from build123d import *

# Parameters (mm, degrees)
SKETCH_1_W          = 35
SKETCH_1_H          = 39
SKETCH_1_R          = 2.1
EXTRUDE_1_DEPTH     = 8
SKETCH_2_R          = 1.6
CUT_EXTRUDE_1_DEPTH = 54.009433123
SKETCH_5_R          = 6
EXTRUDE_3_DEPTH     = 8
M4X0_7_1_D          = 3.3


with BuildPart() as part:
    # 草图1 → 凸台-拉伸1 (new body)
    with BuildSketch(Plane.XY):
        with Locations((17.5, 19.5)):
            Rectangle(SKETCH_1_W, SKETCH_1_H)
        with Locations((17.5, 23.5)):
            Circle(SKETCH_1_R, mode=Mode.SUBTRACT)
    extrude(amount=EXTRUDE_1_DEPTH)

    # 草图2 → 切除-拉伸1 (cut, through all)
    with BuildSketch(Plane(origin=(0, 39, 0), x_dir=(1, 0, 0), z_dir=(0, 1, 0))):
        with Locations(Location((5, -4, 0), (0, 0, 270))):
            Circle(SKETCH_2_R)
        with Locations(Location((30, -4, 0), (0, 0, 270))):
            Circle(SKETCH_2_R)
    extrude(amount=-CUT_EXTRUDE_1_DEPTH, mode=Mode.SUBTRACT)

    # 草图5 → 凸台-拉伸3 (add)
    with BuildSketch(Plane.XY.offset(8)):
        with BuildLine():
            Line((35, 39), (59.879399185, 32.179773011))
            ThreePointArc((59.879399185, 32.179773011), (66.424469933, 24.663544764), (62.025315767, 15.720442351))
            Line((62.025315767, 15.720442351), (35, 0))
            Line((35, 0), (35, 39))
        make_face()
        with Locations((57.5, 23.5)):
            Circle(SKETCH_5_R, mode=Mode.SUBTRACT)
    extrude(amount=-EXTRUDE_3_DEPTH)

    # M4x0.7 螺纹孔1 (through all)
    with Locations(Plane(origin=(0, 39, 0), x_dir=(1, 0, 0), z_dir=(0, 1, 0))):
        with Locations((5, -4), (30, -4)):
            Hole(M4X0_7_1_D / 2)


solid = part.part
CAD build for the part. Positions are in the model's coordinates, mm. Round coordinates to 2 decimals unless told otherwise and drop trailing zeros. Order: outer loops, then holes, each group sorted by start corner. A loop starts at its lowest first (then second) coordinate and runs counter-clockwise, first axis right, second up. Notation, with made-up numbers: (18, 13) -> (47, 13) arc R16 ccw to (47, 30) -> close; hole circle Ø7 at (58, 26.5). An arc over 180 degrees is marked (long way). Write each question's results on one line, items separated by ' | '.
1. Wall check: line 1 along X through (y, z) = (11.5, 4); line 2 along X through (y, z) = (21, 3.5); line 3 along X through (y, z) = (19.5, 4). Give the ranges that are in metal, low to high. Write a range as [from, to].
Findings below:
line 1: x = [0, 3.35], [6.65, 28.35], [31.65, 54.77] | line 2: x = [0, 3.43], [6.57, 28.43], [31.57, 52.05], [62.95, 66.15] | line 3: x = [0, 3.35], [6.65, 28.35], [31.65, 53.03], [61.97, 65.56]
2. Cut at D-D (x = 30). Give the cut face in (y, z).
Findings below:
outline: (0, 0) -> (39, 0) -> (39, 2.35) -> (0, 2.35) -> close; (0, 5.65) -> (39, 5.65) -> (39, 8) -> (0, 8) -> close
3. Cut at B-B (x = 17.5). Give the cut face in (y, z).
Findings below:
outline: (0, 0) -> (21.4, 0) -> (21.4, 8) -> (0, 8) -> close; (25.6, 0) -> (39, 0) -> (39, 8) -> (25.6, 8) -> close
4. Cut at C-C (y = 14). Give the cut face in (x, z).
Findings below:
outline: (0, 0) -> (59.07, 0) -> (59.07, 8) -> (0, 8) -> close; hole circle Ø3.3 at (5, 4); hole circle Ø3.3 at (30, 4)
5. Cut at A-A (z = 4). Give the cut face in (x, y), plus the area to 3 significant figures.
Findings below:
outline: (0, 0) -> (3.35, 0) -> (3.35, 39) -> (0, 39) -> close; (6.65, 0) -> (28.35, 0) -> (28.35, 39) -> (6.65, 39) -> close; (31.65, 0) -> (35, 0) -> (62.03, 15.72) arc R9 ccw to (59.88, 32.18) -> (35, 39) -> (31.65, 39) -> close; hole circle Ø4.2 at (17.5, 23.5); hole circle Ø12 at (57.5, 23.5) | area: 1,770 mm²
6. Flat gauge pins, fed straight in: P1, Ø8, axis at x = 55.5, y = 11.5, coming from the -Z side; P2, Ø3, axis at y = 16.5, z = 2.5, coming from the +X side; P3, Ø3.5, axis at x = 17.5, y = 23.5, coming from the -Z side. Where does each tip first touch, or does it go through?
Findings below:
P1: stops at z = 0 | P2: stops at x = 64.62 | P3: passes through
7. Pull direction X, two halves, no side cores. Call faces 1 (the face through (31.31, 19.23, 5)), 2 (the face through (26, 20, 8)), 3 (the face through (48.7, 7.97, 4.06)): pulls with the +X half, pulls with the -X half, needs draft (parallel to the pull), parting line crosses it, or undercut.
Findings below:
face 1: undercut | face 2: needs draft | face 3: pulls with the +X half
